Can you work these out from the model? Positions are in its coordinate system, mm. A direction names the side the tool comes from. Give positions to 0.01 mm unless a question says otherwise; leave off trailing zeros. Answer in a Markdown table with one row per item.
from build123d import *

# Parameters (mm, degrees)
SKETCH2_R           = 6.35
CUT_EXTRUDE1_DEPTH  = 127.301164781
SKETCH3_R           = 25.4
SKETCH3_R_2         = 12.7
CUT_EXTRUDE3_DEPTH  = 127.301164781
SKETCH4_R           = 5.715
CUT_EXTRUDE4_DEPTH  = 127.301164781
SKETCH5_R           = 6.35
SKETCH5_R_2         = 5.715
SKETCH5_R_3         = 12.7
SKETCH5_R_4         = 25.4
BOSS_EXTRUDE1_DEPTH = 12.065


with BuildPart() as part:
    # Sketch1 → Revolve2 (revolve)
    with BuildSketch(Plane.XY, mode=Mode.PRIVATE) as revolve2_sk:
        with BuildLine():
            ThreePointArc((88.9, 7.747), (86.0425, 4.8895), (88.9, 2.032))
            Line((88.9, 2.032), (88.9, 0))
            Line((88.9, 0), (76.2, 0))
            Line((76.2, 0), (76.2, 2.54))
            Line((76.2, 2.54), (69.85, 2.54))
            Line((69.85, 2.54), (69.85, 0))
            Line((69.85, 0), (0, 0))
            Line((0, 0), (0, 12.065))
            Line((0, 12.065), (80.01, 12.065))
            Line((80.01, 12.065), (80.01, 10.795))
            Line((80.01, 10.795), (86.36, 10.795))
            Line((86.36, 10.795), (86.36, 12.065))
            Line((86.36, 12.065), (88.9, 12.065))
            Line((88.9, 12.065), (88.9, 7.747))
        make_face()
    revolve(revolve2_sk.sketch.rotate(Axis((0, 28.20697446, 0), (0, -1, 0)), 90), axis=Axis((0, 28.20697446, 0), (0, -1, 0)))

    # Sketch2 → Cut-Extrude1 (cut, through all)
    with BuildSketch(Plane(origin=(0, 12.065, 0), x_dir=(1, 0, 0), z_dir=(0, 1, 0))):
        with Locations(Location((-25.4, -47.752, 0), (0, 0, 270))):
            Circle(SKETCH2_R)
        with Locations(Location((25.4, -47.752, 0), (0, 0, 270))):
            Circle(SKETCH2_R)
    extrude(amount=-CUT_EXTRUDE1_DEPTH, mode=Mode.SUBTRACT)

    # Sketch3 → Cut-Extrude3 (cut, through all)
    with BuildSketch(Plane(origin=(0, 12.065, 0), x_dir=(1, 0, 0), z_dir=(0, 1, 0))):
        with Locations(Location((0, 38.1, 0), (0, 0, 270))):
            Circle(SKETCH3_R)
        with Locations(Location((25.4, 0, 0), (0, 0, 270))):
            Circle(SKETCH3_R_2)
        with Locations(Location((-25.4, 0, 0), (0, 0, 270))):
            Circle(SKETCH3_R_2)
    extrude(amount=-CUT_EXTRUDE3_DEPTH, mode=Mode.SUBTRACT)

    # Sketch4 → Cut-Extrude4 (cut, through all)
    with BuildSketch(Plane(origin=(0, 12.065, 0), x_dir=(1, 0, 0), z_dir=(0, 1, 0))):
        with Locations(Location((50.8, -25.4, 0), (0, 0, 270))):
            Circle(SKETCH4_R)
        with Locations(Location((50.8, 25.4, 0), (0, 0, 270))):
            Circle(SKETCH4_R)
        with Locations(Location((-50.8, -25.4, 0), (0, 0, 270))):
            Circle(SKETCH4_R)
        with Locations(Location((-50.8, 25.4, 0), (0, 0, 270))):
            Circle(SKETCH4_R)
    extrude(amount=-CUT_EXTRUDE4_DEPTH, mode=Mode.SUBTRACT)

    # Sketch5 → Boss-Extrude1 (add, through all)
    with BuildSketch(Plane(origin=(0, 12.065, 0), x_dir=(1, 0, 0), z_dir=(0, 1, 0))):
        with Locations((-25.4, -47.752)):
            Circle(SKETCH5_R)
        with Locations((-50.8, -25.4)):
            Circle(SKETCH5_R_2)
        with Locations((-25.4, 0)):
            Circle(SKETCH5_R_3)
        with Locations((0, 38.1)):
            Circle(SKETCH5_R_4)
        with Locations((-50.8, 25.4)):
            Circle(SKETCH5_R_2)
        with Locations((50.8, 25.4)):
            Circle(SKETCH5_R_2)
        with Locations((25.4, 0)):
            Circle(SKETCH5_R_3)
        with Locations((25.4, -47.752)):
            Circle(SKETCH5_R)
        with Locations((50.8, -25.4)):
            Circle(SKETCH5_R_2)
    extrude(amount=-BOSS_EXTRUDE1_DEPTH)


solid = part.part
Q1. On a 3-axis mill with a long thin cutter (end or side, diameter ignored), from which of +Z, -Z, +X, -X, +Y, -Y can I reach the whole of each face in a straight line? I mean faces 5 (the face through (62, 2.54, 34)), 6 (the face through (-24.033, 11.421, 76.315)), 7 (the face through (-1, 0, -1)). Say none if no direction works.
Checked values:
| item | result |
|---|---|
| face 5 | -Y |
| face 6 | +Y |
| face 7 | +Z, -Z, +X, -X, -Y |
Q2. If I drill on line 1 (X direction, y = 0.85, z = 0); line 2 (X direction, y = 11.5, z = -19); line 3 (Z direction, x = -61.5, y = 1.75), over which ranges is the centre line in solid material (lowest first)? Write a range as [from, to].
Checked values:
| item | result |
|---|---|
| line 1 | x = [-88.9, -76.2], [-69.85, 69.85], [76.2, 88.9] |
| line 2 | x = [-86.85, -84.24], [-77.72, 77.72], [84.24, 86.85] |
| line 3 | z = [-64.19, -44.99], [-33.12, 33.12], [44.99, 64.19] |
Q3. For pin 1 (3 mm diameter, centred on y = 6.5, z = -62, fed in from -X); pin 2 (3 mm diameter, centred on x = 3.5, y = 6, fed in from +Z); pin 3 (1 mm diameter, centred on y = 2, z = 33.5, fed in from +X), each with a flat end and sliding along its axis, tell me the tip position at first contact or that it passes through.
Checked values:
| item | result |
|---|---|
| pin 1 | stops at x = -64.51 |
| pin 2 | stops at z = 87.67 |
| pin 3 | stops at x = 82.55 |
Q4. If we mould it in two halves opening along X, with no side actions, what happens to faces 1 (the face through (-60.083, 1.002, -65.523)), 2 (the face through (74.388, 1.288, -16.519)), 3 (the face through (68.2, 1.3, -15.1)), 4 (the face through (-39.9, 0, 65.4))? For each: released by +X, released by -X, zero draft, split by the parting line, or undercut.
Checked values:
| item | result |
|---|---|
| face 1 | split by the parting line |
| face 2 | undercut |
| face 3 | undercut |
| face 4 | zero draft |
